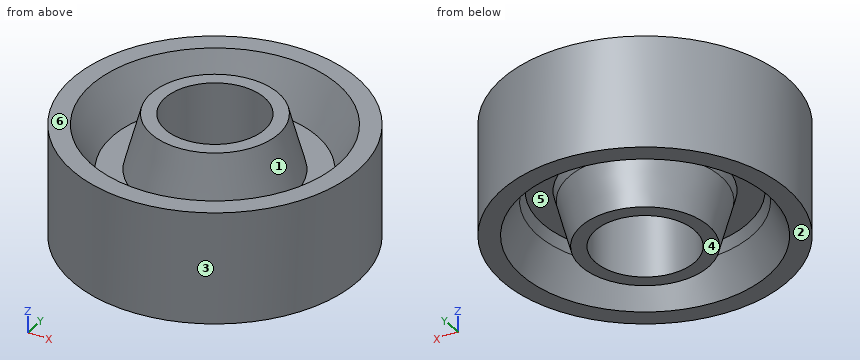
Autodesk Inventor part; units mm, degrees
ref_plane "YZ Plane" through (0, 0, 0) normal (1, 0, 0) x (0, 1, 0)
ref_plane "XZ Plane" through (0, 0, 0) normal (0, 1, 0) x (-1, 0, 0)
ref_plane "XY Plane" through (0, 0, 0) normal (0, 0, 1) x (1, 0, 0)
sketch "Sketch1" plane through (0, 0, 0) normal (1, 0, 0) x (0, 1, 0)
  line L0 (0, 0) -> (0, -43)
  line L1 (0, -43) -> (4.5, -43)
  line L2 (0, 0) -> (4.5, 0)
  line L3 (4.5, 0) -> (0, 0)
  line L4 (0, 0) -> (30, 0)
  line L5 (30, 0) -> (25.5, 0)
  line L6 (25.5, 0) -> (30, 0)
  line L7 (30, 0) -> (30, -3.5)
  line L8 (30, -3.5) -> (30, -39.5)
  line L9 (30, -39.5) -> (30, -43)
  line L10 (23.7723, -3.5) -> (30, -3.5)
  line L11 (30, -39.5) -> (23.7723, -39.5)
  line L12 (23.7723, -39.5) -> (18.5312, -28.2604)
  line L13 (23.7723, -39.5) -> (36.1738, -39.5) construction
  line L14 (4.5, -43) -> (8.4495, -28.2604)
  line L15 (4.5, -43) -> (19.7596, -43) construction
  line L16 (0, 0) -> (0, -21.5)
  line L17 (0, -21.5) -> (30, -21.5)
  line L18 (18.5312, -28.2604) -> (17.0108, -25)
  line L19 (0, -21.5) -> (0, -21.5)
  line L20 (0, -21.5) -> (0, -25)
  line L21 (0, -25) -> (0, -18)
  line L22 (9.3236, -25) -> (17.0108, -25)
  line L23 (23.7723, -3.5) -> (17.0108, -18)
  line L24 (17.0108, -18) -> (9.3236, -18)
  line L25 (9.3236, -18) -> (4.5, 0)
  line L26 (9.3236, -25) -> (8.2254, -29.0967)
  line L27 (0, -43) -> (-16, -43)
  line L28 (-16, -43) -> (-16, -23.25)
  dimension "d0" = 43
  dimension "d1" = 4.5
  dimension "d2" = 4.5
  dimension "d3" = 30
  dimension "d4" = 4.5
  dimension "d5" = 3.5
  dimension "d6" = 36
  dimension "d7" = 3.5
  dimension "d8" = 115
  dimension "d9" = 75
  dimension "d11" = 21.5
  dimension "d12" = 0
  dimension "d13" = 3.5
  dimension "d14" = 7
  dimension "d29" = 25
  dimension "d30" = 25
  dimension "d31" = 15.006
  dimension "d32" = 15.001
  dimension "d33" = 14.5
  dimension "d34" = 3.5
  dimension "d35" = 4.8516
  dimension "d36" = 23.0242
  dimension "d37" = 15.4786
  dimension "d38" = 6.1738
  dimension "d39" = 10.2404
  dimension "d40" = 16
sketch "Sketch2" plane through (0, 0, 0) normal (0, 1, 0) x (-1, 0, 0)
  point P0 (0, 0)
sketch "Sketch3" plane through (0, 0, 0) normal (1, 0, 0) x (0, 1, 0)
  line L0 (-16, -42.9893) -> (-16, -42.9893)
  line L1 (0, 0) -> (0, -42.9893)
  line L2 (0, -42.9893) -> (-16, -42.9893)
  dimension "d16" = 0
sketch "Sketch4" plane through (0, 0, 0) normal (1, 0, 0) x (0, 1, 0)
  line L0 (-16, 5.5421) -> (-16, 5.5421)
  line L1 (-16, -17.3048) -> (-16, -42.7531)
  point P0 (0, 0)
  dimension "d17" = 0
revolve "Revolution1" add sketch "Sketch1" angle 360 about axis through (0, -16, -43) along (0, 0, 1) contours L2 L25 L24 L23 L10 L8 L17 L0 | L17 L8 L11 L12 L18 L22 L26 L14 L1 L0
properties material "Iron, Cast"
Read the model definition and answer for the solid it produces. Units are mm, in the model's axes. Face numbers are marked on the shaded views. A direction names the side the tool comes from. Give positions to 0.01 mm unless a question says otherwise; leave off trailing zeros. Loops run counter-clockwise (first coordinate to the right, second up) from the corner with the lowest first, then second, coordinate; pieces in that order, holes last.
Item 1: Each of these flat-tipped pins is pushed along its axis until it touches: pin 1 Ø10 at (y, z) = (-18, -14.5) entering from -X; pin 2 Ø12 at (x, y) = (36, -38) entering from -Z; pin 3 Ø12 at (y, z) = (-31.5, -5.5) entering from -X. Where does it stop, or does it pass through?
Item 2: The part is cut by section C-C (x = 0). Write down the section's boundary in (y, z), and give its area (3 significant figures).
Item 3: The part is cut by section D-D (z = -7). Write down the section's boundary in (x, y), and give its area (3 significant figures).
Item 4: The part is cut by section B-B (z = -23.5). Write down the section's boundary in (x, y), and give its area (3 significant figures).
Item 5: The part is cut by section A-A (y = -16). Write down the section's boundary in (x, z), and give its area (3 significant figures).
Item 6: The mould has two halves that part along Y. Classify the marked faces 1, 2 and 3: released by +Y, released by -Y, zero draft, split by the parting line, or undercut.
Item 7: Find the intervals of material crossed by line 1 along Y through (x, z) = (-19.5, -5); line 2 along Y through (x, z) = (0, -10); line 3 along X through (y, z) = (2, -13.5), in increasing order.
Item 8: For the marked faces 4, 5 and 6, determine the directions among +Z, -Z, +X, -X, +Y, -Y from which every point of the face is accessible in a straight line to the end or side of a thin tool.
Taken from the geometry:
1. pin 1: stops at x = -46
1. pin 2: stops at z = -39.5
1. pin 3: stops at x = -45.01
2. outline: (-62, -39.5) - (-55.77, -39.5) - (-50.53, -28.26) - (-49.01, -25) - (-41.32, -25) - (-40.45, -28.26) - (-36.5, -43) - (-32, -43) - (-32, 0) - (-36.5, 0) - (-41.32, -18) - (-49.01, -18) - (-55.77, -3.5) - (-62, -3.5) - close; (0, -43) - (4.5, -43) - (8.45, -28.26) - (9.32, -25) - (17.01, -25) - (18.53, -28.26) - (23.77, -39.5) - (30, -39.5) - (30, -3.5) - (23.77, -3.5) - (17.01, -18) - (9.32, -18) - (4.5, 0) - (0, 0) - close
2. area: 1,470 mm2
3. outline: circle Ø92 at (0, -16); circle Ø44.75 at (0, -16); hole circle Ø76.28 at (0, -16); hole circle Ø32 at (0, -16)
3. area: 2,850 mm2
4. outline: circle Ø92 at (0, -16); hole circle Ø32 at (0, -16)
4. area: 5,840 mm2
5. outline: (-46, -39.5) - (-39.77, -39.5) - (-34.53, -28.26) - (-33.01, -25) - (-25.32, -25) - (-24.45, -28.26) - (-20.5, -43) - (-16, -43) - (-16, 0) - (-20.5, 0) - (-25.32, -18) - (-33.01, -18) - (-39.77, -3.5) - (-46, -3.5) - close; (16, -43) - (20.5, -43) - (24.45, -28.26) - (25.32, -25) - (33.01, -25) - (34.53, -28.26) - (39.77, -39.5) - (46, -39.5) - (46, -3.5) - (39.77, -3.5) - (33.01, -18) - (25.32, -18) - (20.5, 0) - (16, 0) - close
5. area: 1,470 mm2
6. face 1: undercut
6. face 2: zero draft
6. face 3: split by the parting line
7. line 1: y = -57.66 to -49.86, -25.84 to -6.16, 17.86 to 25.66
7. line 2: y = -62 to -52.74, -39.18 to -32, 0 to 7.18, 20.74 to 30
7. line 3: x = -42.33 to -30.14, -16.05 to 16.05, 30.14 to 42.33
8. face 4: -Z, +X, -X, +Y, -Y
8. face 5: -Z
8. face 6: +Z
